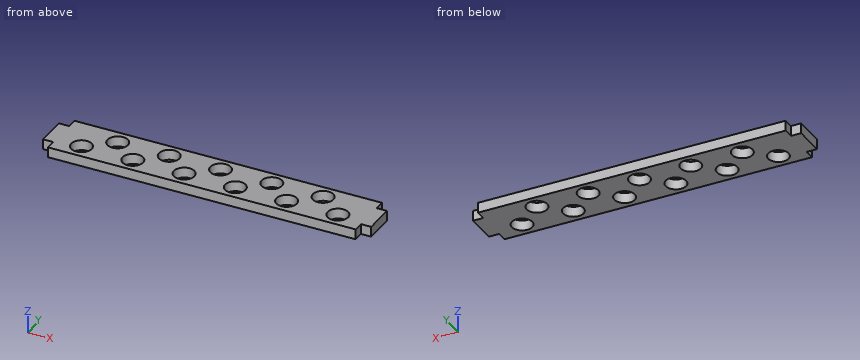
```python
from build123d import *

# Parameters (mm, degrees)
F0_R     = 10
F0_W     = 10
F0_H     = 30
F1_DEPTH = 10


with BuildPart() as f1:
    # F0 (on Top) → F1 (new body)
    with BuildSketch(Plane.XY):
        Polygon((-245.196861, 22.822646), (54.803139, 22.822646), (54.803139, 32.822646), (54.803139, 62.822646), (54.803139, 72.822646), (-245.196861, 72.822646), (-245.196861, 62.822646), (-245.196861, 32.822646), align=None)
        with Locations((-220.196861, 37.822646)):
            Circle(F0_R, mode=Mode.SUBTRACT)
        with Locations((-170.196861, 37.822646)):
            Circle(F0_R, mode=Mode.SUBTRACT)
        with Locations((-120.196861, 37.822646)):
            Circle(F0_R, mode=Mode.SUBTRACT)
        with Locations((-70.196861, 37.822646)):
            Circle(F0_R, mode=Mode.SUBTRACT)
        with Locations((-20.196861, 37.822646)):
            Circle(F0_R, mode=Mode.SUBTRACT)
        with Locations((29.803139, 37.822646)):
            Circle(F0_R, mode=Mode.SUBTRACT)
        with Locations((-195.196861, 57.822646)):
            Circle(F0_R, mode=Mode.SUBTRACT)
        with Locations((-145.196861, 58.276102)):
            Circle(F0_R, mode=Mode.SUBTRACT)
        with Locations((-95.196861, 58.276102)):
            Circle(F0_R, mode=Mode.SUBTRACT)
        with Locations((-45.196861, 58.276102)):
            Circle(F0_R, mode=Mode.SUBTRACT)
        with Locations((4.803139, 58.276102)):
            Circle(F0_R, mode=Mode.SUBTRACT)
        with Locations((-250.196861, 47.822646)):
            Rectangle(F0_W, F0_H)
        with Locations((59.803139, 47.822646)):
            Rectangle(F0_W, F0_H)
    extrude(amount=F1_DEPTH)


solid = f1.part
```
Geometry: final body of the model. Coordinates: model frame, mm. Coordinates: 2 decimals unless noted, no trailing zeros. Order: outer loops, then holes, each group sorted by start corner. A loop starts at its lowest first (then second) coordinate and runs counter-clockwise, first axis right, second up. Notation, with made-up numbers: (10.25, 32.5) -> (38.25, 32.5) arc R26 cw to (38.25, 64.5) -> close; hole circle Ø7 at (-40, 68). An arc over 180 degrees is marked (long way). Write each question's results on one line, items separated by ' | '. Start each with the question number.
1) Cut plane C-C, the plane z = 8.5. State how many separate pieces and enclosed holes the cut face has, and give its area (3 significant figures).
2) Material intervals for line 1 along Y through (x, z) = (-220.5, 0.5); line 2 along Y through (x, z) = (-171, 1.5); line 3 along X through (y, z) = (54, 2.75), sorted ascending.
3) Cut plane B-B, the plane x = -14. Output: boundary loops of the cut face in (y, z).
4) Cut plane D-D, the plane x = -51. Output: boundary loops of the cut face in (y, z).
5) First-contact query: pin 1 (3 mm diameter, centred on x = 57.5, z = 6.5, fed in from -Y); pin 2 (5 mm diameter, centred on y = 28.5, z = 7, fed in from -X); pin 3 (3 mm diameter, centred on x = 60.5, z = 4, fed in from +Y). Flat tips, straight axial feed; report the tip coordinate or a pass-through.
6) Cut plane A-A, the plane y = 52. Output: boundary loops of the cut face in (x, z).
Checks:
1) separate pieces: 1 | enclosed holes: 11 | area: 12,100 mm^2
2) line 1: 22.82 to 27.83, 47.82 to 72.82 | line 2: 22.82 to 27.85, 47.79 to 72.82 | line 3: -255.2 to -204.44, -185.96 to -154.24, -136.16 to -104.24, -86.16 to -54.24, -36.16 to -4.24, 13.84 to 64.8
3) outline: (22.82, 0) -> (29.97, 0) -> (29.97, 10) -> (22.82, 10) -> close; (45.67, 0) -> (72.82, 0) -> (72.82, 10) -> (45.67, 10) -> close
4) outline: (22.82, 0) -> (50.13, 0) -> (50.13, 10) -> (22.82, 10) -> close; (66.42, 0) -> (72.82, 0) -> (72.82, 10) -> (66.42, 10) -> close
5) pin 1: y = 32.82 | pin 2: x = -245.2 | pin 3: y = 62.82
6) outline: (-255.2, 0) -> (-203.33, 0) -> (-203.33, 10) -> (-255.2, 10) -> close; (-187.07, 0) -> (-152.98, 0) -> (-152.98, 10) -> (-187.07, 10) -> close; (-137.41, 0) -> (-102.98, 0) -> (-102.98, 10) -> (-137.41, 10) -> close; (-87.41, 0) -> (-52.98, 0) -> (-52.98, 10) -> (-87.41, 10) -> close; (-37.41, 0) -> (-2.98, 0) -> (-2.98, 10) -> (-37.41, 10) -> close; (12.59, 0) -> (64.8, 0) -> (64.8, 10) -> (12.59, 10) -> close
